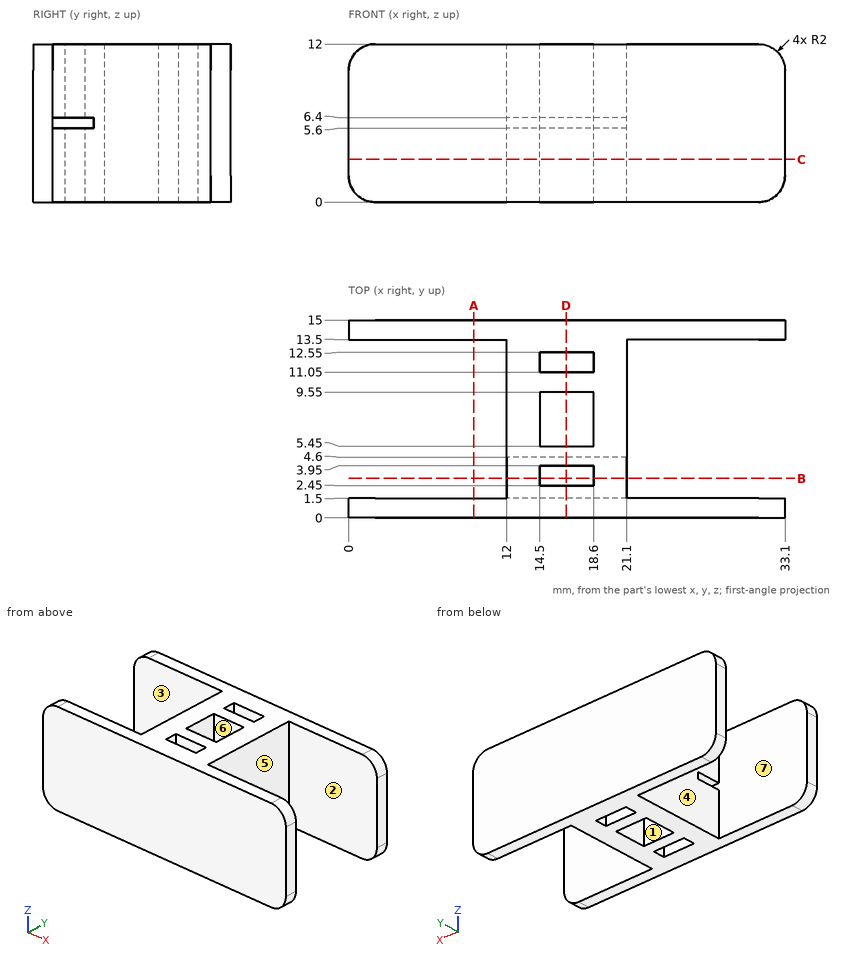
The drawing under review shows one solid part. Ordinate dimensions are in mm from its lowest x, y, z. A direction names the side the tool comes from. Coordinates: 2 decimals unless noted, no trailing zeros. Loops run counter-clockwise (first coordinate to the right, second up) from the corner with the lowest first, then second, coordinate; pieces in that order, holes last.
Item 1: Clearance check with flat-ended pins moving along their axes: pin 1 (4.5 mm diameter, centred on y = 6.5, z = 3, fed in from -X); pin 2 (4.5 mm diameter, centred on y = 7.5, z = 5.5, fed in from +X). State where each tip first meets the part, or that it passes through.
Completed:
pin 1: stops at x = 12
pin 2: stops at x = 21.1
Item 2: Add section A-A (x = 9.5). Write out the cut boundary in (y, z).
Completed:
outline: (0, 0) - (1.5, 0) - (1.5, 12) - (0, 12) - close; (13.5, 0) - (15, 0) - (15, 12) - (13.5, 12) - close
Item 3: Add section D-D (x = 16.5). Write out the cut boundary in (y, z), and give its area (3 significant figures).
Completed:
outline: (0, 0) - (2.45, 0) - (2.45, 5.6) - (1.5, 5.6) - (1.5, 6.4) - (2.45, 6.4) - (2.45, 12) - (0, 12) - close; (3.95, 0) - (5.45, 0) - (5.45, 12) - (3.95, 12) - (3.95, 6.4) - (4.6, 6.4) - (4.6, 5.6) - (3.95, 5.6) - close; (9.55, 0) - (11.05, 0) - (11.05, 12) - (9.55, 12) - close; (12.55, 0) - (15, 0) - (15, 12) - (12.55, 12) - close
area: 93.5 mm2
Item 4: Add section C-C (z = 3.25). Write out the cut boundary in (x, y), and give its area (3 significant figures).
Completed:
outline: (0, 0) - (33.1, 0) - (33.1, 1.5) - (21.1, 1.5) - (21.1, 13.5) - (33.1, 13.5) - (33.1, 15) - (0, 15) - (0, 13.5) - (12, 13.5) - (12, 1.5) - (0, 1.5) - close; hole (14.5, 2.45) - (18.6, 2.45) - (18.6, 3.95) - (14.5, 3.95) - close; hole (14.5, 5.45) - (18.6, 5.45) - (18.6, 9.55) - (14.5, 9.55) - close; hole (14.5, 11.05) - (18.6, 11.05) - (18.6, 12.55) - (14.5, 12.55) - close
area: 179 mm2
Item 5: Add section B-B (y = 3). Write out the cut boundary in (x, z).
Completed:
outline: (12, 0) - (14.5, 0) - (14.5, 5.6) - (12, 5.6) - close; (12, 6.4) - (14.5, 6.4) - (14.5, 12) - (12, 12) - close; (18.6, 0) - (21.1, 0) - (21.1, 5.6) - (18.6, 5.6) - close; (18.6, 6.4) - (21.1, 6.4) - (21.1, 12) - (18.6, 12) - close
Item 6: For the marked faces 1, 2 and 3, list the 3-axis set-ups (+Z, -Z, +X, -X, +Y, -Y) from which the entire face can be reached by the end or side of a thin tool; tool diameter is ignored.
Completed:
face 1: +Z, -Z
face 2: +Z, -Z, +X
face 3: +Z, -Z, -X
Item 7: Wall thickness on L1, parallel to Y at x = 18, z = 6.5; L2, parallel to X at y = 6.75, z = 8.5; L3, parallel to Y at x = 28.5, z = 10: over which ranges is each line inside the solid? List them lowest first.
Completed:
L1: y = 0 to 2.45, 3.95 to 5.45, 9.55 to 11.05, 12.55 to 15
L2: x = 12 to 14.5, 18.6 to 21.1
L3: y = 0 to 1.5, 13.5 to 15
Item 8: Draft analysis for pull direction X (two halves, no side actions). For the marked faces 4, 5, 6 and 7, state which applies: pulls with the +X half, pulls with the -X half, needs draft (parallel to the pull), parting line crosses it, or undercut.
Completed:
face 4: pulls with the -X half
face 5: pulls with the +X half
face 6: undercut
face 7: needs draft
